```python
from build123d import *

# Parameters (mm, degrees)
PAD_DEPTH    = 20
SKETCH001_R  = 2.15
POCKET_DEPTH = 47
CHAMFER_SIZE = 1.5


with BuildPart() as part:
    # Sketch → Pad (new body)
    with BuildSketch(Plane.XZ):
        with BuildLine():
            Line((4.039009, 42.574694), (2.655848, 42.793836))
            ThreePointArc((2.906222, 44.374125), (1.990891, 43.709168), (2.655848, 42.793836))
            Line((2.906222, 44.374125), (5.030423, 44.037575))
            Line((5.030423, 44.037575), (5.030423, 45.679508))
            ThreePointArc((6.630423, 45.679508), (5.830423, 46.479508), (5.030423, 45.679508))
            Line((6.630423, 45.679508), (6.630423, 44.166555))
            Line((6.630423, 44.166555), (8.44155, 45.411155))
            Line((8.44155, 45.411155), (9.447306, 46.1366))
            ThreePointArc((10.36219, 44.864349), (10.54179, 45.958576), (9.447306, 46.1366))
            Line((10.36219, 44.864349), (7.849046, 43.062615))
            Line((7.849046, 43.062615), (5.639009, 41.543887))
            Line((5.639009, 41.543887), (7.054906, 39.48349))
            Line((7.054906, 39.48349), (12.329523, 43.108185))
            Line((12.329523, 43.108185), (38.948379, 4.372717))
            Line((134.880474, 70.296864), (38.948379, 4.372717))
            Line((119.305612, 92.961233), (134.880474, 70.296864))
            Line((134.96463, 103.722048), (119.305612, 92.961233))
            Line((142.044114, 93.420062), (134.96463, 103.722048))
            Line((237.976209, 159.344209), (142.044114, 93.420062))
            Line((219.852732, 185.717293), (237.976209, 159.344209))
            Line((225.127349, 189.341989), (219.852732, 185.717293))
            Line((223.711452, 191.402386), (225.127349, 189.341989))
            Line((218.436835, 187.77769), (223.711452, 191.402386))
            Line((218.436835, 187.77769), (217.530661, 189.096345))
            Line((217.530661, 189.096345), (221.384849, 191.744926))
            Line((221.384849, 191.744926), (219.379319, 192.170864))
            ThreePointArc((219.628617, 193.344683), (218.917058, 192.882422), (219.379319, 192.170864))
            Line((219.628617, 193.344683), (221.24827, 193.000698))
            Line((221.24827, 193.000698), (222.339521, 195.334027))
            ThreePointArc((223.426518, 194.825661), (223.137203, 195.623343), (222.339521, 195.334027))
            Line((223.426518, 194.825661), (222.458309, 192.755421))
            Line((222.458309, 192.755421), (225.35977, 192.535103))
            Line((225.35977, 192.535103), (227.205855, 189.8487))
            Line((227.205855, 189.8487), (225.162842, 186.850988))
            Line((225.162842, 186.850988), (229.879355, 185.690134))
            ThreePointArc((229.592563, 184.524909), (230.318572, 184.964126), (229.879355, 185.690134))
            Line((229.592563, 184.524909), (227.449372, 185.052402))
            Line((227.449372, 185.052402), (226.943935, 182.66136))
            ThreePointArc((225.77104, 182.655995), (226.359652, 182.185457), (226.943935, 182.66136))
            Line((225.77104, 182.655995), (226.273638, 185.03361))
            Line((226.273638, 185.03361), (223.79734, 183.331907))
            Line((223.79734, 183.331907), (226.006139, 180.117688))
            Line((226.006139, 180.117688), (232.18733, 184.365377))
            Line((232.18733, 184.365377), (247.106338, 153.120807))
            Line((247.106338, 153.120807), (245.375605, 151.931453))
            Line((226.996861, 139.301656), (245.375605, 151.931453))
            Line((222.409356, 145.977343), (226.996861, 139.301656))
            Line((225.54116, 148.129505), (222.409356, 145.977343))
            Line((229.222491, 142.772473), (225.54116, 148.129505))
            Line((232.271879, 144.868), (229.222491, 142.772473))
            Line((227.910918, 151.214023), (232.271879, 144.868))
            Line((214.971623, 142.322192), (227.910918, 151.214023))
            Line((219.332585, 135.976169), (214.971623, 142.322192))
            Line((222.381972, 138.071696), (219.332585, 135.976169))
            Line((218.700641, 143.428729), (222.381972, 138.071696))
            Line((220.348959, 144.561446), (218.700641, 143.428729))
            Line((224.936464, 137.885759), (220.348959, 144.561446))
            Line((216.560272, 132.129674), (224.936464, 137.885759))
            Line((214.12493, 135.673557), (216.560272, 132.129674))
            Line((214.12493, 135.673557), (161.513364, 99.519102))
            Line((161.513364, 99.519102), (229.635216, 0.388931))
            Line((290.622974, 42.299471), (229.635216, 0.388931))
            Line((294.258763, 37.008711), (290.622974, 42.299471))
            Line((296.31916, 38.424607), (294.258763, 37.008711))
            Line((292.460363, 44.039886), (296.31916, 38.424607))
            Line((292.460363, 44.039886), (293.779018, 44.94606))
            Line((293.779018, 44.94606), (296.611353, 40.824476))
            Line((296.611353, 40.824476), (297.055734, 42.735476))
            ThreePointArc((298.27896, 42.451029), (297.809571, 43.204865), (297.055734, 42.735476))
            Line((298.27896, 42.451029), (297.79847, 40.384748))
            Line((297.79847, 40.384748), (300.094356, 39.873139))
            ThreePointArc((299.821203, 38.647342), (300.570678, 39.123664), (300.094356, 39.873139))
            Line((299.821203, 38.647342), (297.765407, 39.10545))
            Line((297.765407, 39.10545), (296.952983, 36.433452))
            Line((296.952983, 36.433452), (295.39148, 35.360393))
            Line((295.39148, 35.360393), (291.873432, 36.02126))
            Line((291.873432, 36.02126), (290.627867, 32.242369))
            ThreePointArc((289.412187, 32.33524), (289.983665, 31.812832), (290.627867, 32.242369))
            Line((289.412187, 32.33524), (290.101718, 34.427194))
            Line((290.101718, 34.427194), (287.564776, 35.169274))
            ThreePointArc((287.653171, 36.393701), (287.114763, 35.817166), (287.564776, 35.169274))
            Line((287.653171, 36.393701), (290.071377, 35.686353))
            Line((290.071377, 35.686353), (288.237588, 38.354863))
            Line((288.237588, 38.354863), (285.035062, 36.129048))
            Line((285.035062, 36.129048), (289.282752, 29.947856))
            Line((289.282752, 29.947856), (228.604015, -5.17314))
            Line((37.917178, -1.189353), (228.604015, -5.17314))
            Line((9.169934, 31.108727), (37.917178, -1.189353))
            Line((15.351126, 35.356416), (9.169934, 31.108727))
            Line((13.142327, 38.570636), (15.351126, 35.356416))
            Line((10.619339, 36.836849), (13.142327, 38.570636))
            Line((12.456819, 36.836849), (10.619339, 36.836849))
            ThreePointArc((12.456819, 35.236849), (13.256819, 36.036849), (12.456819, 36.836849))
            Line((10.207431, 35.236849), (12.456819, 35.236849))
            Line((10.207431, 33.941322), (10.207431, 35.236849))
            ThreePointArc((8.607431, 33.941322), (9.407431, 33.141322), (10.207431, 33.941322))
            Line((8.607431, 37.271491), (8.607431, 33.941322))
            Line((5.406588, 38.350772), (8.607431, 37.271491))
            Line((4.039009, 40.340858), (5.406588, 38.350772))
            Line((4.039009, 40.340858), (4.039009, 42.574694))
        make_face()
        Polygon((43.567429, 2.693476), (225.814584, -1.113991), (165.579391, 86.539602), align=None, mode=Mode.SUBTRACT)
    extrude(amount=PAD_DEPTH)

    # Sketch001 (on DatumPlane) → Pocket (cut)
    with BuildSketch(Plane(origin=(-5.122749, 0, 7.454568), x_dir=(-0.824159, 0, -0.566359), z_dir=(-0.566359, 0, 0.824159))):
        with Locations((-160.5, 9.989038)):
            Circle(SKETCH001_R)
    extrude(amount=-POCKET_DEPTH, mode=Mode.SUBTRACT)

    # Chamfer
    chamfer_edges = [part.edges().sort_by_distance(p)[0] for p in [
        (128.926695, -9.989038, 99.572803),
    ]]
    chamfer(chamfer_edges, length=CHAMFER_SIZE)


solid = part.part
```
Geometry: final body of the model. Coordinates: model frame, mm. A direction names the side the tool comes from. Coordinates: 2 decimals unless noted, no trailing zeros. Order: outer loops, then holes, each group sorted by start corner. A loop starts at its lowest first (then second) coordinate and runs counter-clockwise, first axis right, second up. Notation, with made-up numbers: (24.25, 62) - (55.25, 62) arc R12 cw to (55.25, 67) - close; hole circle Ø11 at (71.25, 53.5). An arc over 180 degrees is marked (long way). Return JSON: item names as keys, results as strings. Group by question number.
1. Pin query (flat end, axial travel): pin 1 (2 mm diameter, centred on x = 12, y = -11, fed in from +Z); pin 2 (2.5 mm diameter, centred on x = 11, y = -10.5, fed in from -Z); pin 3 (2.5 mm diameter, centred on y = -13.5, z = 35.5, fed in from -X). Return the tip coordinate at first contact, or that it passes through.
2. Pull-direction query (X, two-part tool) for faces 1 (the face through (239.542, -9.86, 168.962)), 2 (the face through (126.984, -9.86, 81.788)), 3 (the face through (105.427, -9.86, 45.203)); classes: pulls with the +X half, pulls with the -X half, needs draft (parallel to the pull), parting line crosses it, or undercut.
3. Cut plane B-B (x = 205.5). Output: boundary loops of the cut face in (y, z).
4. Set-up query: faces 4 (the face through (138.554, -9.86, 98.499)), 5 (the face through (138.15, -10.08, 86.15)), 6 (the face through (185, 0, 59)), 7 (the face through (217.183, -9.86, 139.105)), 8 (the face through (220.69, -9.86, 134.97)). Return all of +Z, -Z, +X, -X, +Y, -Y with unobstructed straight access to the full face (end or side cutting, diameter ignored); none if empty.
5. Cut plane A-A (z = 20). Output: boundary loops of the cut face in (x, y).
6. Material intervals for line 1 along Z through (x, y) = (217.5, -17.75); line 2 along Z through (x, y) = (203.5, -3); line 3 along Z through (x, y) = (215.5, -8.5), sorted ascending. Write a range as [from, to].
7. Cut plane C-C (z = 62). Output: boundary loops of the cut face in (x, y), plus the area to 3 significant figures.
8. Cut plane D-D (x = 86). Output: boundary loops of the cut face in (y, z), plus the area to 3 significant figures.
Resolved:
{
 "1": {"pin 1": "stops at z = 43.11", "pin 2": "stops at z = 27.65", "pin 3": "stops at x = 8.61"},
 "2": {"face 1": "pulls with the +X half", "face 2": "pulls with the -X half", "face 3": "undercut"},
 "3": {"outline": "(-20, -4.69) - (0, -4.69) - (0, -0.69) - (-20, -0.69) - close; (-20, 28.45) - (0, 28.45) - (0, 35.51) - (-20, 35.51) - close; (-20, 129.75) - (0, 129.75) - (0, 137.03) - (-20, 137.03) - close"},
 "4": {"face 4": "+Z, +Y, -Y", "face 5": "none", "face 6": "+Z, -Z, +X, -X, +Y", "face 7": "+Y, -Y", "face 8": "+X, +Y, -Y"},
 "5": {"outline": "(19.06, -20) - (28.21, -20) - (28.21, 0) - (19.06, 0) - close; (61.69, -20) - (68.75, -20) - (68.75, 0) - (61.69, 0) - close; (211.31, -20) - (216.16, -20) - (216.16, 0) - (211.31, 0) - close; (258.17, -20) - (272.1, -20) - (272.1, 0) - (258.17, 0) - close"},
 "6": {"line 1": "z = [-4.94, -0.94], [10.99, 18.05], [132.78, 138.64], [144.06, 145.27]", "line 2": "z = [-4.65, -0.65], [31.36, 38.42], [128.37, 135.65]", "line 3": "z = [-4.9, -0.9], [13.9, 20.96], [133.67, 141.55], [142.69, 143.9]"},
 "7": {"outline": "(122.81, -20) - (129.87, -20) - (129.87, 0) - (122.81, 0) - close; (182.44, -20) - (187.3, -20) - (187.3, 0) - (182.44, 0) - close", "area": "238 mm²"},
 "8": {"outline": "(-20, -2.19) - (0, -2.19) - (0, 1.81) - (-20, 1.81) - close; (-20, 31.85) - (0, 31.85) - (0, 36.71) - (-20, 36.71) - close", "area": "177 mm²"}
}
